from build123d import *

# Parameters (mm, degrees)
F0_W     = 10.8331
F0_H     = 4.3942
F1_DEPTH = 12.7
F2_SIZE  = 1.905
F3_R     = 3.175
F4_DEPTH = 25.4


with BuildPart() as f1:
    # F0 (on Front) → F1 (new body)
    with BuildSketch(Plane.XZ):
        with Locations((5.41655, 2.1971)):
            Rectangle(F0_W, F0_H)
    extrude(amount=F1_DEPTH)

    # F2
    f2_edges = [f1.edges().sort_by_distance(p)[0] for p in [
        (10.8331, -6.35, 4.3942),
        (0, -6.35, 4.3942),
    ]]
    chamfer(f2_edges, length=F2_SIZE)

    # F3 (on face) → F4 (cut)
    with BuildSketch(Plane(origin=(0, 0, 0), x_dir=(1, 0, 0), z_dir=(0, 0, -1))):
        with Locations((5.41655, 6.35)):
            Circle(F3_R)
    extrude(amount=-F4_DEPTH, mode=Mode.SUBTRACT)


solid = f1.part
Can you work these out from the model? Positions are in its coordinate system, mm. Give positions to 0.01 mm unless a question says otherwise; leave off trailing zeros. Loops run counter-clockwise (first coordinate to the right, second up) from the corner with the lowest first, then second, coordinate; pieces in that order, holes last. Notation, with made-up numbers: (-13.5, 5) -> (-5.5, 5) arc R25 ccw to (-5.5, 39) -> close; hole circle Ø9 at (-4.5, 62.25). An arc over 180 degrees is marked (long way). Return JSON: item names as keys, results as strings.
Q1. I want a section at A-A, the plane y = -6.35. List the corners of the cut face in (x, z) for me (3 decimals), then the cut area to 3 significant figures.
Checks:
{"outline": "(0, 0) -> (2.242, 0) -> (2.242, 4.394) -> (1.905, 4.394) -> (0, 2.489) -> close; (8.592, 0) -> (10.833, 0) -> (10.833, 2.489) -> (8.928, 4.394) -> (8.592, 4.394) -> close", "area": "16.1 mm2"}
Q2. I want a section at C-C, the plane x = 3.25. List the corners of the cut face in (y, z) for me, then the cut area to 3 significant figures.
Checks:
{"outline": "(-12.7, 0) -> (-8.67, 0) -> (-8.67, 4.39) -> (-12.7, 4.39) -> close; (-4.03, 0) -> (0, 0) -> (0, 4.39) -> (-4.03, 4.39) -> close", "area": "35.4 mm2"}
Q3. I want a section at D-D, the plane y = -1. List the corners of the cut face in (x, z) for me (3 decimals), then the cut area to 3 significant figures.
Checks:
{"outline": "(0, 0) -> (10.833, 0) -> (10.833, 2.489) -> (8.928, 4.394) -> (1.905, 4.394) -> (0, 2.489) -> close", "area": "44.0 mm2"}
Q4. I need wall thicknesses on probe 1 along X at (y, z) = (-6.35, 1.05); probe 2 along X at (y, z) = (-6.35, 2.95); probe 3 along Y at (x, z) = (2.5, 2.7). Which ranges of each line are inside material? Lowest first, please.
Checks:
{"probe 1": "x = 0 to 2.24, 8.59 to 10.83", "probe 2": "x = 0.46 to 2.24, 8.59 to 10.37", "probe 3": "y = -12.7 to -7.6, -5.1 to 0"}
Q5. For pin 1 Ø1 at (y, z) = (-5.5, 3.5) entering from +X, with a flat end and sliding along its axis, tell me the tip position at first contact or that it passes through.
Checks:
{"pin 1": "stops at x = 10.32"}
Q6. We'd pull the mould along Y, two halves only. Please class faces 1 (the face through (4, -3, 0)), 2 (the face through (5, 0, 2)), 3 (the face through (5.003, -9.498, 2.166)): released by +Y, released by -Y, zero draft, split by the parting line, or undercut.
Checks:
{"face 1": "zero draft", "face 2": "released by +Y", "face 3": "undercut"}
Q7. I want a section at B-B, the plane z = 1.95. List the corners of the cut face in (x, y) for me (3 decimals), then the cut area to 3 significant figures.
Checks:
{"outline": "(0, -12.7) -> (10.833, -12.7) -> (10.833, 0) -> (0, 0) -> close; hole circle Ø6.35 at (5.417, -6.35)", "area": "106 mm2"}
